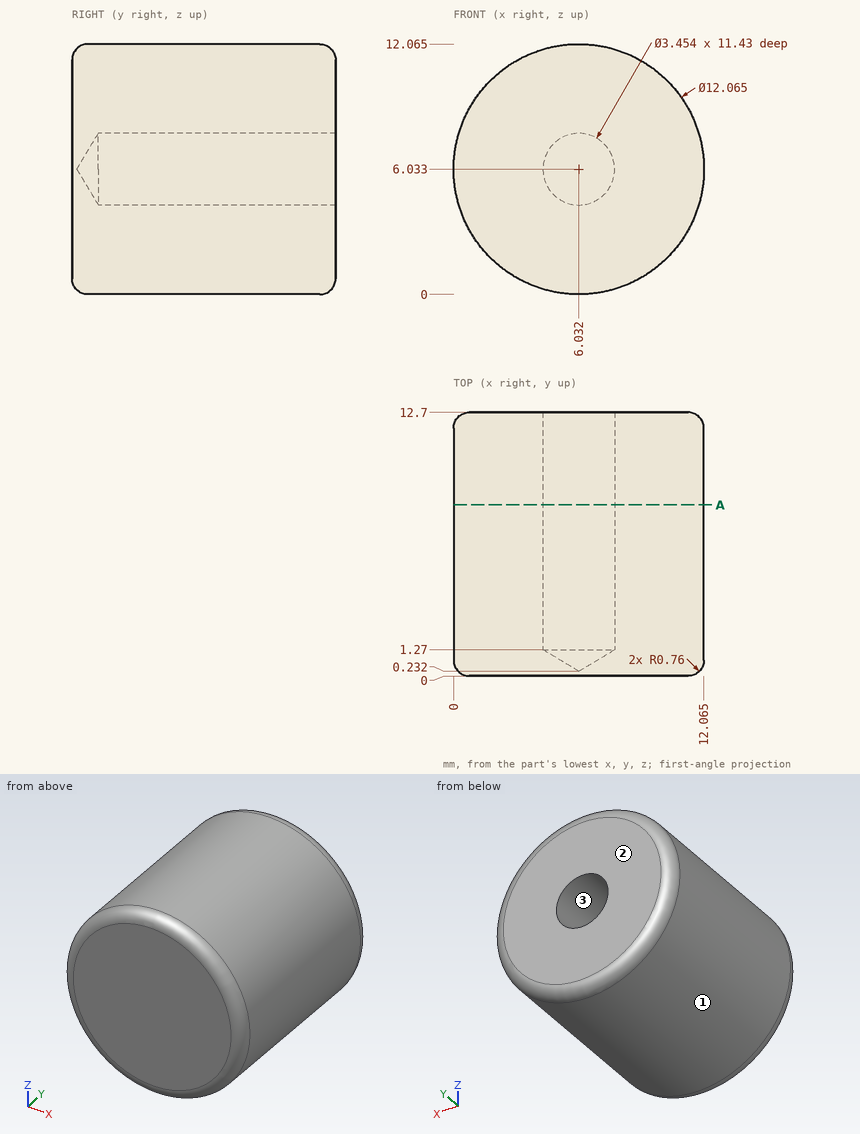
For this review, use the dimensioned drawing (mm, ordinates from the lowest corner) and the shaded views. Coordinates: 2 decimals unless noted, no trailing zeros. Loops run counter-clockwise (first coordinate to the right, second up) from the corner with the lowest first, then second, coordinate; pieces in that order, holes last. Notation, with made-up numbers: (68, 85.5) -> (78, 85.5) arc R24 cw to (78, 100.5) -> close; hole circle Ø5 at (-36, -35.75). An arc over 180 degrees is marked (long way). Return JSON: item names as keys, results as strings. Group by question number.
(1) Consider section A-A, the plane y = 8.25. Give the boundary of the cut face in (x, z) (1 decimal).
(2) Mouldability with a two-part tool opening along X and no side actions: class the marked faces 1, 2 and 3 as pulls with the +X half, pulls with the -X half, needs draft (parallel to the pull), parting line crosses it, or undercut.
(3) For pin 1 Ø2 at (x, z) = (6.03, 6.03) entering from +Y (1 decimal); pin 2 Ø1 at (y, z) = (9.5, 10) entering from -X (1 decimal); pin 3 Ø1.5 at (y, z) = (4.5, 1.5) entering from +X, all flat-tipped, find the tip position at first contact; note any pin that passes through.
(4) To check wall thickness, follow L1, parallel to X at y = 4, z = 7.5 (1 decimal); L2, parallel to X at y = 3.5, z = 7.25 (1 decimal); L3, parallel to Z at x = 6.25, y = 7 (1 decimal). State the ranges of each line that lie inside material, in increasing order.
Results below:
{
 "1": {"outline": "circle Ø12.1 at (6, 6); hole circle Ø3.5 at (6, 6)"},
 "2": {"face 1": "parting line crosses it", "face 2": "needs draft", "face 3": "undercut"},
 "3": {"pin 1": "stops at y = 0.8", "pin 2": "stops at x = 1.1", "pin 3": "stops at x = 10.73"},
 "4": {"L1": "x = 0.2 to 5.1, 6.9 to 11.9", "L2": "x = 0.1 to 4.8, 7.3 to 11.9", "L3": "z = 0 to 4.3, 7.7 to 12.1"}
}
